```python
from build123d import *

# Parameters (mm, degrees)
SKETCH_1_W          = 20
SKETCH_1_H          = 63
EXTRUDE_1_DEPTH     = 5
HOLE_WIZARD_M3_1_D  = 3.4
FILLET_1_R          = 5
CUT_EXTRUDE_1_DEPTH = 10
FILLET_2_R          = 1.1


with BuildPart() as part:
    # 草图1 → 凸台-拉伸1 (new body)
    with BuildSketch(Plane(origin=(0, 0, 0), x_dir=(0, 0, -1), z_dir=(1, 0, 0))):
        with Locations((10, 31.5)):
            Rectangle(SKETCH_1_W, SKETCH_1_H)
    extrude(amount=EXTRUDE_1_DEPTH)

    # M3 间隙孔1 (through all)
    with Locations(Plane(origin=(5, 0, 0), x_dir=(0, 0, -1), z_dir=(1, 0, 0))):
        with Locations((3, 11), (17, 11), (16, 60.25), (4, 60.25)):
            Hole(HOLE_WIZARD_M3_1_D / 2)

    # 圆角1
    fillet_1_edges = [part.edges().sort_by_distance(p)[0] for p in [
        (2.5, 63, 0),
        (2.5, 63, -20),
        (2.5, 0, -20),
        (2.5, 0, 0),
    ]]
    fillet(fillet_1_edges, radius=FILLET_1_R)

    # 草图4 → 切除-拉伸1 (cut)
    with BuildSketch(Plane(origin=(5, 0, 0), x_dir=(0, 0, -1), z_dir=(1, 0, 0))):
        Polygon((2.5, 45.855823048), (17.5, 55), (2.5, 55), align=None)
        Polygon((17.5, 40), (17.5, 49.144176952), (2.5, 40), align=None)
        Polygon((17.5, 25.855823048), (17.5, 35), (2.5, 35), align=None)
        Polygon((17.5, 20), (2.5, 29.144176952), (2.5, 20), align=None)
    extrude(amount=-CUT_EXTRUDE_1_DEPTH, mode=Mode.SUBTRACT)

    # 圆角2
    fillet_2_edges = [part.edges().sort_by_distance(p)[0] for p in [
        (2.5, 55, -17.5),
        (2.5, 45.855823048, -2.5),
        (2.5, 55, -2.5),
        (2.5, 40, -2.5),
        (2.5, 49.144176952, -17.5),
        (2.5, 40, -17.5),
        (2.5, 25.855823048, -17.5),
        (2.5, 35, -2.5),
        (2.5, 35, -17.5),
        (2.5, 20, -17.5),
        (2.5, 20, -2.5),
        (2.5, 29.144176952, -2.5),
    ]]
    fillet(fillet_2_edges, radius=FILLET_2_R)


solid = part.part
```
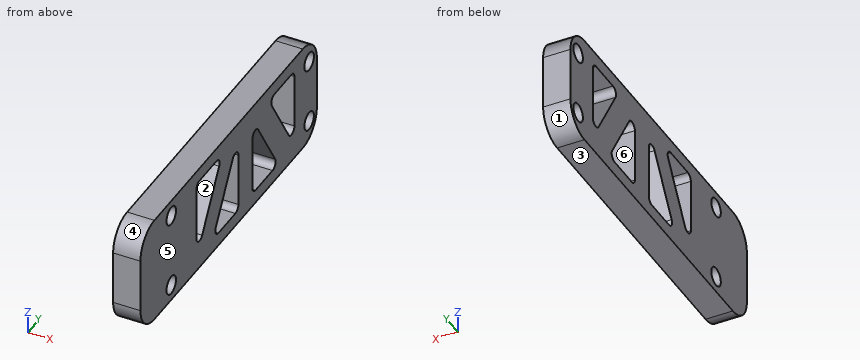
Model file for the job. Use its own axes, mm. Face numbers are marked on the shaded views. A direction names the side the tool comes from. Give positions to 0.01 mm unless a question says otherwise; leave off trailing zeros. Loops run counter-clockwise (first coordinate to the right, second up) from the corner with the lowest first, then second, coordinate; pieces in that order, holes last. Notation, with made-up numbers: M 36.5,36 L 93.5,36 A24 ccw 93.5,49 Z; hole C 7,30 d10. An arc over 180 degrees is marked long. Use one line per item in the form item = value.
Item 1: Flat gauge pins, fed straight in: pin 1 Ø2 at (x, z) = (2.5, -16.5) entering from +Y; pin 2 Ø5 at (y, z) = (39, -15.5) entering from -X. Where does each tip first touch, or does it go through?
Filled in:
pin_1 = 62.97
pin_2 = 0
Item 2: Which spindle directions (+Z, -Z, +X, -X, +Y, -Y) get a long thin tool onto all of the face, cutting with end or side? Do the marked faces 1 and 2. Say none if no direction does.
Filled in:
face_1 = -Z, +X, -X, +Y
face_2 = +X, -X
Item 3: Two-plate mould, pull along Z, no slides. Class the marked faces 3, 4, 5 and 6: released by +Z, released by -Z, zero draft, split by the parting line, or undercut.
Filled in:
face_3 = released by -Z
face_4 = released by +Z
face_5 = zero draft
face_6 = undercut
Item 4: Slice it at A-A on y = 11. List the corners of the cut face in (x, z), and give its area (3 significant figures).
Filled in:
outline = M 0,-20 L 5,-20 L 5,-18.7 L 0,-18.7 Z; M 0,-15.3 L 5,-15.3 L 5,-4.7 L 0,-4.7 Z; M 0,-1.3 L 5,-1.3 L 5,0 L 0,0 Z
area = 66.0 mm^2
Item 5: Slice it at D-D on y = 60.25. List the corners of the cut face in (x, z), and give its area (3 significant figures).
Filled in:
outline = M 0,-19.47 L 5,-19.47 L 5,-17.7 L 0,-17.7 Z; M 0,-14.3 L 5,-14.3 L 5,-5.7 L 0,-5.7 Z; M 0,-2.3 L 5,-2.3 L 5,-0.53 L 0,-0.53 Z
area = 60.7 mm^2
Item 6: Slice it at C-C on z = -12. List the corners of the cut face in (x, y).
Filled in:
outline = M 0,0 L 5,0 L 5,20 L 0,20 Z; M 0,23.35 L 5,23.35 L 5,29.21 L 0,29.21 Z; M 0,35 L 5,35 L 5,40 L 0,40 Z; M 0,45.79 L 5,45.79 L 5,51.65 L 0,51.65 Z; M 0,55 L 5,55 L 5,63 L 0,63 Z
Item 7: Slice it at B-B on x = 0.8. Give the number of separate pieces and of enclosed holes in the cut face, and give its area (3 significant figures).
Filled in:
separate_pieces = 1
enclosed_holes = 8
area = 943 mm^2
Item 8: Drill centre lines: L1, parallel to Y at x = 1.6, z = -14.25; L2, parallel to Y at x = 1.3, z = -4; L3, parallel to Z at x = 3.5, y = 12.5. Where is each one in solid material? Low to high.
Filled in:
L1 = 0 to 20.23, 21.97 to 27.84, 35 to 40, 47.16 to 53.03, 54.77 to 63
L2 = 0.1 to 9.63, 12.37 to 20, 28.21 to 46.79, 55 to 58.55, 61.95 to 62.9
L3 = -20 to -17.8, -16.2 to -3.8, -2.2 to 0
